```python
from build123d import *

# Parameters (mm, degrees)
F0_W     = 12.7
F0_H     = 16.2401907146
F1_DEPTH = 3.81
F2_W     = 12.7
F2_H     = 3.81
F3_DEPTH = 12.7
F4_R     = 1.27
F5_DEPTH = 10.16
F6_W     = 1.6954607129
F6_H     = 8.2879924147
F7_DEPTH = 5.08


with BuildPart() as f1:
    # F0 (on Front) → F1 (new body)
    with BuildSketch(Plane.XZ):
        with Locations((6.35, 8.1200953573)):
            Rectangle(F0_W, F0_H)
        Polygon((-5.7594607129, 37.0478025981), (0, 16.2401907146), (12.7, 16.2401907146), (18.4594607129, 37.0478025981), align=None)
    extrude(amount=F1_DEPTH)

    # F2 (on face) → F3 (join)
    with BuildSketch(Plane.XZ.offset(3.81)):
        with Locations((6.35, 1.905)):
            Rectangle(F2_W, F2_H)
        with Locations((6.35, 7.747)):
            Rectangle(F2_W, F2_H)
    extrude(amount=F3_DEPTH)

    # F4 (on face) → F5 (join)
    with BuildSketch(Plane.XZ.offset(3.81)):
        with Locations((14.5957274362, 33.9156836271)):
            Circle(F4_R)
        with Locations((-1.0984551627, 33.9156836271)):
            Circle(F4_R)
    extrude(amount=F5_DEPTH)

    # F6 (on face) → F7 (join)
    with BuildSketch(Plane.XZ.offset(3.81)):
        with Locations((6.35, 27.3775784299)):
            Rectangle(F6_W, F6_H)
    extrude(amount=F7_DEPTH)


solid = f1.part
```
Here's how the part is built. I have some questions about the finished solid (model axes, mm). A direction names the side the tool comes from. Round coordinates to 2 decimals unless told otherwise and drop trailing zeros. Loops run counter-clockwise (first coordinate to the right, second up) from the corner with the lowest first, then second, coordinate; pieces in that order, holes last.
1. Suppose I cut it at D-D, the plane z = 11. Please give me the cut outline in (x, y).
Answers:
outline: (0, -3.81) - (12.7, -3.81) - (12.7, 0) - (0, 0) - close
2. If I drill on probe 1 along Z at (x, y) = (3.75, -7.75); probe 2 along Z at (x, y) = (14.5, -12.5); probe 3 along Y at (x, z) = (11.25, 20.5), over which ranges is the centre line in solid material (lowest first)?
Answers:
probe 1: z = 0 to 3.81, 5.84 to 9.65
probe 2: z = 32.65 to 35.18
probe 3: y = -3.81 to 0
3. Suppose I cut it at B-B, the plane x = 8.75. Please give me the cut outline in (y, z).
Answers:
outline: (-16.51, 0) - (0, 0) - (0, 37.05) - (-3.81, 37.05) - (-3.81, 9.65) - (-16.51, 9.65) - (-16.51, 5.84) - (-3.81, 5.84) - (-3.81, 3.81) - (-16.51, 3.81) - close
4. Will these pins go through, and if not, where does the flat tip stop? pin 1 (1 mm diameter, centred on x = 9.5, z = 11, fed in from +Y); pin 2 (2 mm diameter, centred on y = -11, z = 24.5, fed in from +X); pin 3 (1.9 mm diameter, centred on x = 6, z = 26.5, fed in from -Y); pin 4 (4 mm diameter, centred on x = 4.5, y = -8, fed in from +Z).
Answers:
pin 1: stops at y = 0
pin 2: passes through
pin 3: stops at y = -8.89
pin 4: stops at z = 31.52
5. Thinking about a two-plate mould opening in Z: for faces 5 (the face through (5.502, -6, 27)), 6 (the face through (6, -8, 0)), 7 (the face through (7, -2, 37.048)), 8 (the face through (6, -6, 23.234)), which applies, released by +Z, released by -Z, zero draft, split by the parting line, or undercut?
Answers:
face 5: zero draft
face 6: released by -Z
face 7: released by +Z
face 8: undercut
6. For faces 1 (the face through (7.198, -6, 27)), 2 (the face through (6, -10, 5.842)), 3 (the face through (0, -6, 6)), 4 (the face through (6, -8.89, 27)), which set-ups out of +Z, -Z, +X, -X, +Y, -Y let a thin tool reach every point of the face, with its end or its side?
Answers:
face 1: +Z, +X, -Y
face 2: +X, -X, -Y
face 3: -Z, -X, +Y, -Y
face 4: +Z, +X, -X, -Y
7. Suppose I cut it at C-C, the plane y = -8. Please give me the cut outline in (x, z).
Answers:
outline: circle Ø2.54 at (-1.1, 33.92); (0, 0) - (12.7, 0) - (12.7, 3.81) - (0, 3.81) - close; (0, 5.84) - (12.7, 5.84) - (12.7, 9.65) - (0, 9.65) - close; (5.5, 23.23) - (7.2, 23.23) - (7.2, 31.52) - (5.5, 31.52) - close; circle Ø2.54 at (14.6, 33.92)
8. Suppose I cut it at A-A, the plane y = -14.75. Please give me the cut outline in (x, z), and give its area (3 significant figures).
Answers:
outline: (0, 0) - (12.7, 0) - (12.7, 3.81) - (0, 3.81) - close; (0, 5.84) - (12.7, 5.84) - (12.7, 9.65) - (0, 9.65) - close
area: 96.8 mm2
